Can you work these out from the model? Positions are in its coordinate system, mm. Round coordinates to 2 decimals unless told otherwise and drop trailing zeros. Loops run counter-clockwise (first coordinate to the right, second up) from the corner with the lowest first, then second, coordinate; pieces in that order, holes last. Notation, with made-up numbers: M -32,82 L 26,82 A31 cw 26,119 Z; hole C 31,-26 d11. An arc over 180 degrees is marked long. Return JSON: item names as keys, results as strings.
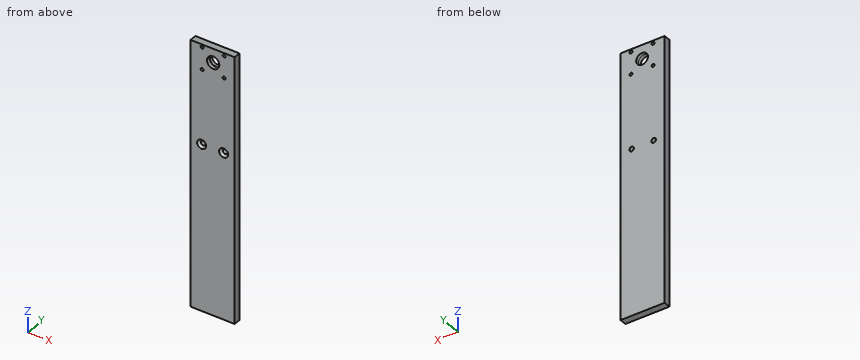
```python
from build123d import *

# Parameters (mm, degrees)
BOSS_EXTRUDE1_DEPTH                             = 76.2
BOSS_EXTRUDE1_DEPTH_BACK                        = 76.2
SKETCH3_W                                       = 50.8
SKETCH3_H                                       = 7.9375
M12_CLEARANCE_HOLE2_D                           = 13.5
CSK_FOR_M5_FLAT_HEAD_MACHINE_SCREW1_D           = 5.3
CSK_FOR_M5_FLAT_HEAD_MACHINE_SCREW1_CSINK_D     = 10.4
CSK_FOR_M5_FLAT_HEAD_MACHINE_SCREW1_CSINK_ANGLE = 90
SKETCH26_W                                      = 50.8
SKETCH26_H                                      = 152.4
BOSS_EXTRUDE2_DEPTH                             = 7.9375
SKETCH27_R                                      = 7.112
CUT_EXTRUDE2_DEPTH                              = 4.318
M3_CLEARANCE_HOLE1_D                            = 3.4
M3_CLEARANCE_HOLE1_DEPTH                        = 15.24
M3_CLEARANCE_HOLE1_TIP                          = 1.021463052


with BuildPart() as part:
    # Sketch3 → Boss-Extrude1 (new, two sides: drawn at the far end of the back side and taken through both)
    with BuildSketch(Plane.XY.offset(-BOSS_EXTRUDE1_DEPTH_BACK)):
        Rectangle(SKETCH3_W, SKETCH3_H)
    extrude(amount=BOSS_EXTRUDE1_DEPTH + BOSS_EXTRUDE1_DEPTH_BACK)

    # M12 Clearance Hole2 (through all)
    with Locations(Plane(origin=(0, 3.96875, 0), x_dir=(1, 0, 0), z_dir=(0, 1, 0))):
        with Locations((0.625840615, -60.325)):
            Hole(M12_CLEARANCE_HOLE2_D / 2)

    # CSK for M5 Flat Head Machine Screw1 (through all)
    with Locations(Plane(origin=(0, -3.96875, 0), x_dir=(-1, 0, 0), z_dir=(0, -1, 0))):
        with Locations((-12.7, 38.1), (12.7, 38.1)):
            CounterSinkHole(CSK_FOR_M5_FLAT_HEAD_MACHINE_SCREW1_D / 2, CSK_FOR_M5_FLAT_HEAD_MACHINE_SCREW1_CSINK_D / 2, counter_sink_angle=CSK_FOR_M5_FLAT_HEAD_MACHINE_SCREW1_CSINK_ANGLE)

    # Sketch26 → Boss-Extrude2 (add)
    with BuildSketch(Plane(origin=(0, 3.96875, 0), x_dir=(1, 0, 0), z_dir=(0, 1, 0))):
        with Locations((0, 152.4)):
            Rectangle(SKETCH26_W, SKETCH26_H)
    extrude(amount=-BOSS_EXTRUDE2_DEPTH)

    # Sketch27 → Cut-Extrude2 (cut)
    with BuildSketch(Plane.XZ.offset(3.96875)):
        with Locations(Location((0.625840615, 60.325, 0), (0, 0, 270))):
            Circle(SKETCH27_R)
    extrude(amount=-CUT_EXTRUDE2_DEPTH, mode=Mode.SUBTRACT)

    # M3 Clearance Hole1
    with Locations(Plane(origin=(0, -3.96875, 0), x_dir=(-1, 0, 0), z_dir=(0, -1, 0))):
        with Locations((-13.325840615, -47.625), (-13.325840615, -73.025), (12.074159385, -73.025), (12.074159385, -47.625)):
            Hole(M3_CLEARANCE_HOLE1_D / 2, depth=M3_CLEARANCE_HOLE1_DEPTH)
            with Locations((0, 0, -(M3_CLEARANCE_HOLE1_DEPTH + M3_CLEARANCE_HOLE1_TIP / 2))):  # 118° drill point
                Cone(0, M3_CLEARANCE_HOLE1_D / 2, M3_CLEARANCE_HOLE1_TIP, mode=Mode.SUBTRACT)


solid = part.part
```
Q1. I'm going to push a flat-ended pin straight in: pin 1 Ø3 at (x, z) = (13.33, 73.03) entering from +Y. Where does the tip first touch, or does it pass through?
Results:
{"pin 1": "passes through"}
Q2. If I drill on line 1 along Z through (x, y) = (3, -1.5); line 2 along Z through (x, y) = (10, -2.25); line 3 along Y through (x, z) = (13, -42.5), over which ranges is the centre line in solid material (lowest first)?
Results:
{"line 1": "z = -228.6 to 53.62, 67.03 to 76.2", "line 2": "z = -228.6 to -40.3, -35.9 to 76.2", "line 3": "y = -3.18 to 3.97"}
Q3. Suppose I cut it at A-A, the plane z = -38.1. Please give me the cut outline in (x, y), plus the area to 3 significant figures.
Results:
{"outline": "M -25.4,-3.97 L -17.9,-3.97 L -15.35,-1.42 L -15.35,3.97 L -25.4,3.97 Z; M -10.05,-1.42 L -7.5,-3.97 L 7.5,-3.97 L 10.05,-1.42 L 10.05,3.97 L -10.05,3.97 Z; M 15.35,-1.42 L 17.9,-3.97 L 25.4,-3.97 L 25.4,3.97 L 15.35,3.97 Z", "area": "306 mm2"}
